```python
from build123d import *

# Parameters (mm, degrees)
BOSS_EXTRUDE1_DEPTH = 405.754616144
SKETCH2_W           = 405.754616144
SKETCH2_H           = 10
CUT_EXTRUDE1_DEPTH  = 11.5
CAVITY1_START       = 240
CAVITY1_OUTLINE_W   = 38.5
CAVITY1_OUTLINE_H   = 405.754616144
CAVITY1_DEPTH       = 2
SKETCH3_W           = 405.754616144
SKETCH3_H           = 10
CUT_EXTRUDE2_DEPTH  = 38.5


# Read off the part's stored shape, not the designer's step: Cavity1
with BuildPart() as part:
    # Sketch1 → Boss-Extrude1 (new body)
    with BuildSketch(Plane(origin=(0, 0, 546.614427926), x_dir=(-1, 0, 0), z_dir=(0, 0, -1))):
        with BuildLine():
            Line((141, 242), (152.5, 242))
            Line((152.5, 242), (152.5, 240))
            Line((152.5, 240), (141, 240))
            Line((141, 240), (141, 230))
            Line((141, 230), (185, 230))
            ThreePointArc((185, 230), (192.071067812, 227.071067812), (195, 220))
            Line((195, 220), (195, 185))
            Line((195, 185), (205, 185))
            Line((205, 185), (205, 203.610753203))
            Line((205, 203.610753203), (207, 203.610753203))
            Line((207, 203.610753203), (207, 185))
            Line((207, 185), (217, 185))
            Line((217, 185), (217, 230))
            ThreePointArc((217, 230), (210.556349186, 245.556349186), (195, 252))
            Line((195, 252), (141, 252))
            Line((141, 252), (141, 242))
        make_face()
    extrude(amount=BOSS_EXTRUDE1_DEPTH)

    # Sketch2 → Cut-Extrude1 (cut)
    with BuildSketch(Plane(origin=(-141, 0, 0), x_dir=(0, 0, -1), z_dir=(1, 0, 0))):
        with Locations((-343.737119854, 247)):
            Rectangle(SKETCH2_W, SKETCH2_H)
    extrude(amount=-CUT_EXTRUDE1_DEPTH, mode=Mode.SUBTRACT)

    # Cavity1 outline → Cavity1 (cut)
    with BuildSketch(Plane(origin=(0, 0, 0), x_dir=(1, 0, 0), z_dir=(0, 1, 0)).offset(CAVITY1_START)):
        with Locations((-171.75, -343.737119854)):
            Rectangle(CAVITY1_OUTLINE_W, CAVITY1_OUTLINE_H)
    extrude(amount=CAVITY1_DEPTH, mode=Mode.SUBTRACT)

    # Sketch3 → Cut-Extrude2 (cut)
    with BuildSketch(Plane(origin=(-152.5, 0, 0), x_dir=(0, 0, -1), z_dir=(1, 0, 0))):
        with Locations((-343.737119854, 247)):
            Rectangle(SKETCH3_W, SKETCH3_H)
    extrude(amount=-CUT_EXTRUDE2_DEPTH, mode=Mode.SUBTRACT)


solid = part.part
```
Part model, mm, in its own coordinate system. A direction names the side the tool comes from. Give positions to 0.01 mm unless a question says otherwise; leave off trailing zeros. Write each loop counter-clockwise with the first axis right and the second up, starting at its lowest first coordinate (ties: lowest second). Pieces come first, ordered by that corner, then holes. Notation, with made-up numbers: (-22, -25.5) -> (30, -25.5) arc R12 ccw to (30, -17.5) -> close; hole circle Ø9 at (7, 40). An arc over 180 degrees is marked (long way). Put each result on its own line as item: value. Start each with the question number.
Item 1: Wall check: L1, parallel to X at y = 198, z = 478.5; L2, parallel to Y at x = -152, z = 288.5; L3, parallel to X at y = 231, z = 212.5. Give the ranges that are in metal, low to high. Write a range as [from, to].
Item 2: Which spindle directions (+Z, -Z, +X, -X, +Y, -Y) get a long thin tool onto all of the face, cutting with end or side? Do faces 5 (the face through (-141, 235, 347)), 6 (the face through (-191, 246, 347)), 7 (the face through (-195, 203, 347)). Say none if no direction does.
Item 3: Pin check, flat tips, straight feed: pin 1 Ø20.5 at (y, z) = (193.5, 310) entering from +X; pin 2 Ø1.6 at (x, z) = (-206, 366.5) entering from -Y; pin 3 Ø25 at (x, z) = (-155, 296) entering from +Y. Stop position of each tip, or through.
Item 4: Cut at A-A (y = 198.5). List the corners of the cut face in (x, z).
Item 5: Pull direction X, two halves, no side cores. Call faces 1 (the face through (-212, 185, 347)), 2 (the face through (-205, 194, 347)), 3 (the face through (-207, 194, 347)), 4 (the face through (-217, 207, 347)): pulls with the +X half, pulls with the -X half, needs draft (parallel to the pull), parting line crosses it, or undercut.
Item 6: Cut at D-D (y = 223.5). List the corners of the cut face in (x, z), then the cut area to 3 significant figures.
Item 7: Cut at C-C (x = -149). List the corners of the cut face in (y, z), then the cut area to 3 significant figures.
Item 8: Cut at B-B (z = 306). List the corners of the cut face in (x, y), then the cut area to 3 significant figures.
Answer list:
1. L1: x = [-217, -207], [-205, -195]
1. L2: y = [230, 240]
1. L3: x = [-216.98, -141]
2. face 5: +Z, -Z, +X, +Y, -Y
2. face 6: +Z, -Z, +X, +Y
2. face 7: +Z, -Z, +X, -Y
3. pin 1: stops at x = -195
3. pin 2: stops at y = 203.61
3. pin 3: stops at y = 240
4. outline: (-217, 140.86) -> (-207, 140.86) -> (-207, 546.61) -> (-217, 546.61) -> close; (-205, 140.86) -> (-195, 140.86) -> (-195, 546.61) -> (-205, 546.61) -> close
5. face 1: needs draft
5. face 2: undercut
5. face 3: undercut
5. face 4: pulls with the -X half
6. outline: (-217, 140.86) -> (-194.37, 140.86) -> (-194.37, 546.61) -> (-217, 546.61) -> close
6. area: 9,180 mm2
7. outline: (230, 140.86) -> (240, 140.86) -> (240, 546.61) -> (230, 546.61) -> close
7. area: 4,060 mm2
8. outline: (-217, 185) -> (-207, 185) -> (-207, 203.61) -> (-205, 203.61) -> (-205, 185) -> (-195, 185) -> (-195, 220) arc R10 cw to (-185, 230) -> (-141, 230) -> (-141, 240) -> (-191, 240) -> (-191, 252) -> (-195, 252) arc R22 ccw to (-217, 230) -> close
8. area: 1,940 mm2
